For this review, use the dimensioned drawing (mm, ordinates from the lowest corner) and the shaded views. A direction names the side the tool comes from. Give positions to 0.01 mm unless a question says otherwise; leave off trailing zeros. Loops run counter-clockwise (first coordinate to the right, second up) from the corner with the lowest first, then second, coordinate; pieces in that order, holes last. Notation, with made-up numbers: M -4,-27 L 15,-27 A17 ccw 15,2 Z; hole C 41,87.25 d6. An arc over 180 degrees is marked long. Use a Markdown table: item, result. Add a question column.
(1) Add section B-B, the plane z = 28. Give the boundary of the cut face in (x, y), then the cut area to 3 significant figures.
(2) Add section D-D, the plane x = 43.5. Give the boundary of the cut face in (y, z).
(3) Insertion check: pin 1 Ø6 at (x, y) = (28, 4) entering from -Z; pin 2 Ø2 at (y, z) = (12.5, 17) entering from +X; pin 3 Ø6 at (x, y) = (13, 17) entering from +Z. Each pin has a flat end and moves straight along its axis. Give the tip position at first contact, or say it passes through.
(4) Draft analysis for pull direction X (two halves, no side actions). For the marked faces 1, 2 and 3, state which applies: pulls with the +X half, pulls with the -X half, needs draft (parallel to the pull), parting line crosses it, or undercut.
(5) For the marked faces 4, 5 and 6, list the 3-axis set-ups (+Z, -Z, +X, -X, +Y, -Y) from which the entire face can be reached by the end or side of a thin tool; tool diameter is ignored.
(6) Add section A-A, the plane y = 10.25. Give the boundary of the cut face in (x, z) (1 decimal).
(7) For probe 1 along Z at (x, y) = (6.5, 23.25); probe 2 along Z at (x, y) = (70, 19.25); probe 3 along Z at (x, y) = (61.5, 11.5) (1 decimal), list the stretches that pass through material, from the lowest coordinate up.
(8) Add section C-C, the plane x = 64. Give the boundary of the cut face in (y, z).
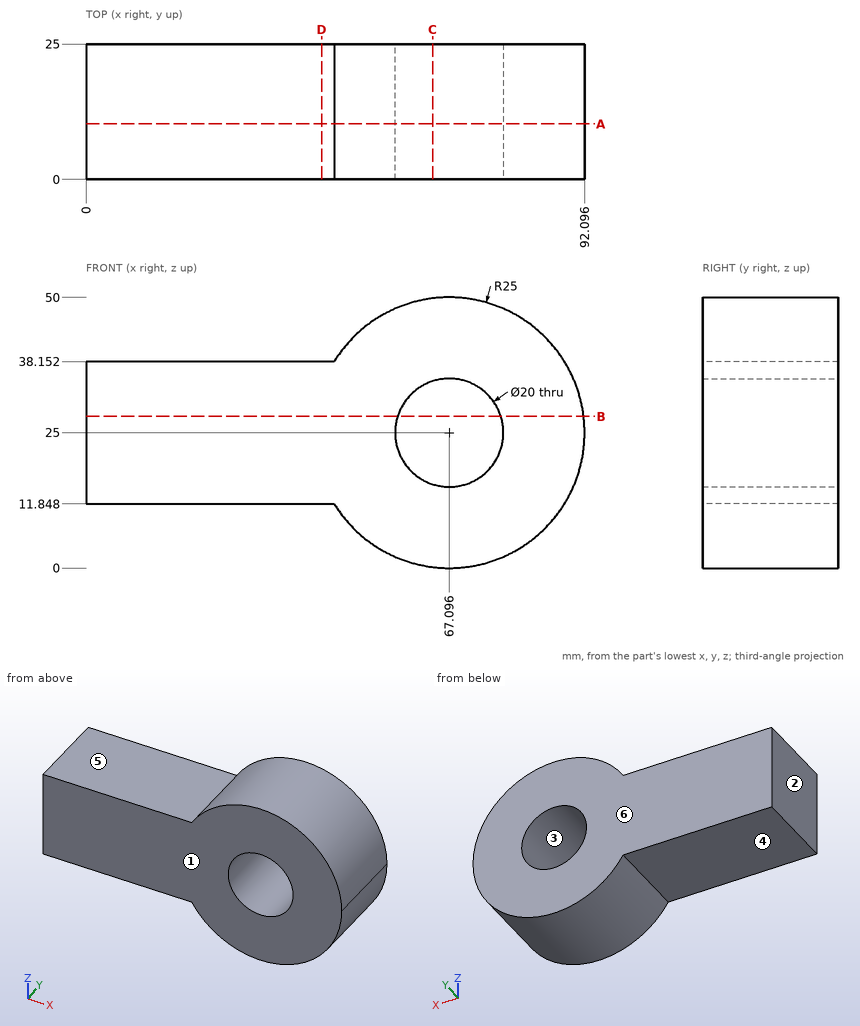
Established:
| question | item | result |
|---|---|---|
| 1 | outline | M 0,0 L 57.56,0 L 57.56,25 L 0,25 Z; M 76.64,0 L 91.92,0 L 91.92,25 L 76.64,25 Z |
| 1 | area | 1,820 mm^2 |
| 2 | outline | M 0,11.85 L 25,11.85 L 25,38.15 L 0,38.15 Z |
| 3 | pin 1 | z = 11.85 |
| 3 | pin 2 | x = 91.1 |
| 3 | pin 3 | z = 38.15 |
| 4 | face 1 | needs draft |
| 4 | face 2 | pulls with the -X half |
| 4 | face 3 | undercut |
| 5 | face 4 | -Z, -X, +Y, -Y |
| 5 | face 5 | +Z, -X, +Y, -Y |
| 5 | face 6 | +Z, -Z, +X, -X, +Y |
| 6 | outline | M 0,11.8 L 45.8,11.8 A25 ccw long 45.8,38.2 L 0,38.2 Z; hole C 67.1,25 d20 |
| 7 | probe 1 | 11.85 to 38.15 |
| 7 | probe 2 | 0.17 to 15.43, 34.57 to 49.83 |
| 7 | probe 3 | 0.6 to 16.7, 33.3 to 49.4 |
| 8 | outline | M 0,0.19 L 25,0.19 L 25,15.49 L 0,15.49 Z; M 0,34.51 L 25,34.51 L 25,49.81 L 0,49.81 Z |
